Build history of the part. All positions in model axes, mm. Face numbers are marked on the shaded views. A direction names the side the tool comes from. Round coordinates to 2 decimals unless told otherwise and drop trailing zeros. Write each loop counter-clockwise with the first axis right and the second up, starting at its lowest first coordinate (ties: lowest second). Pieces come first, ordered by that corner, then holes. Notation, with made-up numbers: (-10.75, -32.5) - (2.25, -32.5) arc R17 ccw to (2.25, -3.5) - close; hole circle Ø8 at (11, 57). An arc over 180 degrees is marked (long way). Answer as a JSON object with one key per item and string values. Group by question number.
Item 1: Probe line 1 (Y direction, x = 22.5, z = 3); line 2 (X direction, y = 6.5, z = 6.5). List the from-to ranges inside material, lowest first. Write a range as from..to.
Item 2: Slice it at B-B, the plane z = 3.5. List the corners of the cut face in (x, y), then the cut area to 3 significant figures.
Item 3: Two-plate mould, pull along Y, no slides. Class the marked faces 1, 2 and 3: +Y half, -Y half, draft (parallel to the pull), parting line (faces both ways), or undercut.
Item 4: Slice it at C-C, the plane y = 2.25. List the corners of the cut face in (x, z).
Item 5: Slice it at A-A, the plane x = -57.5. List the corners of the cut face in (y, z), then the cut area to 3 significant figures.
Item 6: Flat gauge pins, fed straight in: pin 1 (1 mm diameter, centred on y = 1.5, z = 9, fed in from +X); pin 2 (1.2 mm diameter, centred on y = 0.5, z = 6, fed in from +X); pin 3 (2 mm diameter, centred on y = 3.5, z = 9, fed in from +X). Where does each tip first touch, or does it go through?
Item 7: Which spindle directions (+Z, -Z, +X, -X, +Y, -Y) get a long thin tool onto all of the face, cutting with end or side? Do the marked faces 4 and 5. Say none if no direction does.
from build123d import *

# Parameters (mm, degrees)
F1_DEPTH = 10


with BuildPart() as f1:
    # F0 (on Top) → F1 (new body)
    with BuildSketch(Plane.XY):
        with BuildLine():
            Line((-77.5, -10), (74.5, -10))
            ThreePointArc((74.5, -10), (76.62132, -9.12132), (77.5, -7))
            Line((77.5, -7), (77.5, -6.75))
            ThreePointArc((77.5, -6.75), (76.62132, -4.62868), (74.5, -3.75))
            Line((74.5, -3.75), (-64.5, -3.75))
            ThreePointArc((-64.5, -3.75), (-66.62132, -2.87132), (-67.5, -0.75))
            Line((-67.5, -0.75), (-67.5, 0.75))
            ThreePointArc((-67.5, 0.75), (-66.62132, 2.87132), (-64.5, 3.75))
            Line((-64.5, 3.75), (74.5, 3.75))
            ThreePointArc((74.5, 3.75), (76.62132, 4.62868), (77.5, 6.75))
            Line((77.5, 6.75), (77.5, 7))
            ThreePointArc((77.5, 7), (76.62132, 9.12132), (74.5, 10))
            Line((74.5, 10), (-77.5, 10))
            Line((-77.5, 10), (-77.5, -10))
        make_face()
    extrude(amount=F1_DEPTH)


solid = f1.part
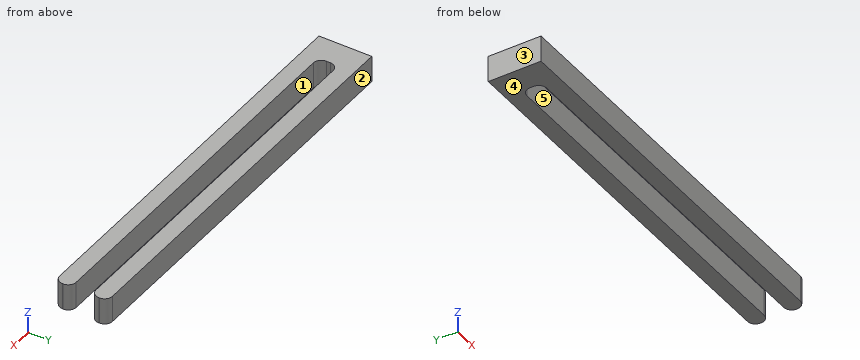
Geometry says:
{
 "1": {"line 1": "y = -10..-3.75, 3.75..10", "line 2": "x = -77.5..77.49"},
 "2": {"outline": "(-77.5, -10) - (74.5, -10) arc R3 ccw to (77.5, -7) - (77.5, -6.75) arc R3 ccw to (74.5, -3.75) - (-64.5, -3.75) arc R3 cw to (-67.5, -0.75) - (-67.5, 0.75) arc R3 cw to (-64.5, 3.75) - (74.5, 3.75) arc R3 ccw to (77.5, 6.75) - (77.5, 7) arc R3 ccw to (74.5, 10) - (-77.5, 10) - close", "area": "2,010 mm^2"},
 "3": {"face 1": "undercut", "face 2": "+Y half", "face 3": "draft"},
 "4": {"outline": "(-77.5, 0) - (-67.1, 0) - (-67.1, 10) - (-77.5, 10) - close"},
 "5": {"outline": "(-10, 0) - (-3.75, 0) - (-3.75, 10) - (-10, 10) - close; (3.75, 0) - (10, 0) - (10, 10) - (3.75, 10) - close", "area": "125 mm^2"},
 "6": {"pin 1": "stops at x = -67.23", "pin 2": "stops at x = -67.48", "pin 3": "stops at x = 76.48"},
 "7": {"face 4": "-Z, +X, -X, +Y, -Y", "face 5": "+Z, -Z, +X"}
}
